Answer from the drawing. Dimensions are ordinates in mm from the lowest x, y and z of the part. A direction names the side the tool comes from. Coordinates: 2 decimals unless noted, no trailing zeros. Loops run counter-clockwise (first coordinate to the right, second up) from the corner with the lowest first, then second, coordinate; pieces in that order, holes last. Notation, with made-up numbers: M 87,55 L 102,55 A27 ccw 102,89 Z; hole C -11,82 d10. An arc over 180 degrees is marked long. Put each result on its own line as item: value.
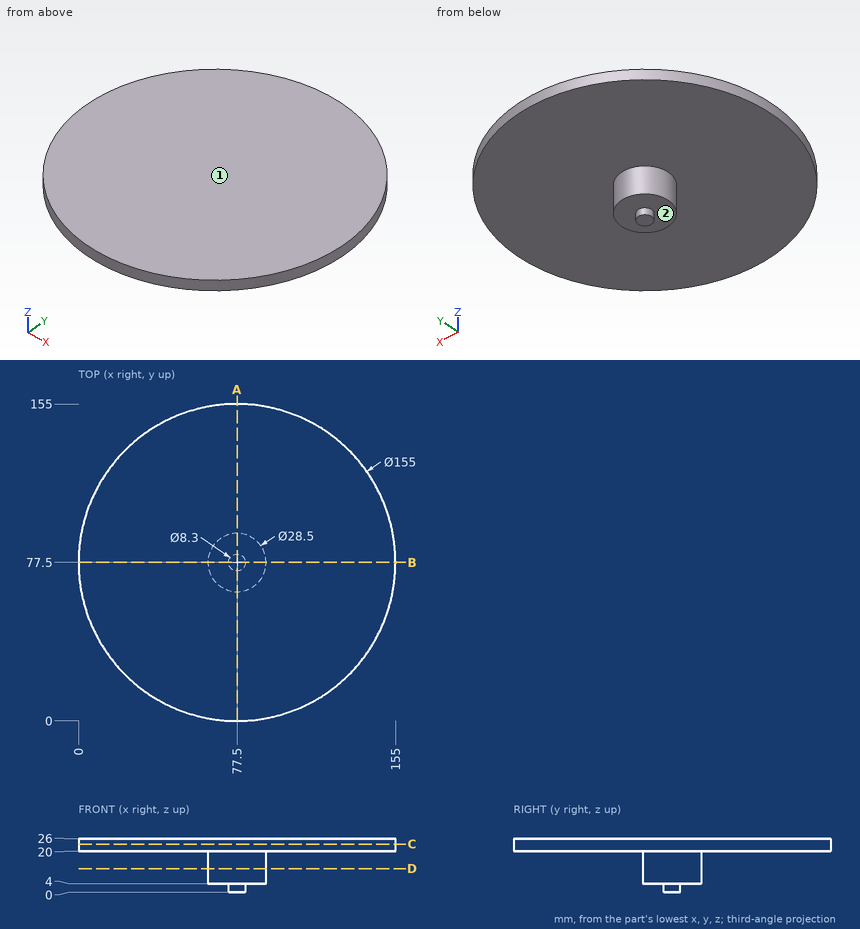
1) Which of the six approach directions +Z, -Z, +X, -X, +Y, -Y give full straight-line access (tool end or side, diameter ignored) to the marked faces 1 and 2?
Answer list:
face 1: +Z, +X, -X, +Y, -Y
face 2: -Z
2) Find section C-C, the plane z = 23.5. Write down the section's boundary in (x, y).
Answer list:
outline: C 77.5,77.5 d155
3) Given pin 1 Ø4 at (x, y) = (135, 120.5) entering from -Z; pin 2 Ø1.5 at (x, z) = (67.5, 22.5) entering from -Y; pin 3 Ø6 at (y, z) = (63, 19.5) entering from -X, each flat-ended and moving along its own axis, determine where each tip first touches the part or whether it passes through.
Answer list:
pin 1: stops at z = 20
pin 2: stops at y = 0.55
pin 3: stops at x = 0.86
4) Straight lines are drawn through the part: line 1 (Z direction, x = 78, y = 88); line 2 (Z direction, x = 105, y = 28); line 3 (X direction, y = 67, z = 18.75). For each, find the intervals that lie inside material, in ascending order. Write a range as [from, to].
Answer list:
line 1: z = [4, 26]
line 2: z = [20, 26]
line 3: x = [67.87, 87.13]
5) Find section D-D, the plane z = 11.5. Write down the section's boundary in (x, y), plus the area to 3 significant figures.
Answer list:
outline: C 77.5,77.5 d28.5
area: 638 mm^2
6) Find section A-A, the plane x = 77.5. Write down the section's boundary in (y, z), plus the area to 3 significant figures.
Answer list:
outline: M 0,20 L 63.25,20 L 63.25,4 L 73.35,4 L 73.35,0 L 81.65,0 L 81.65,4 L 91.75,4 L 91.75,20 L 155,20 L 155,26 L 0,26 Z
area: 1,420 mm^2
